Verification items for this drawing (mm, ordinates from the low corner). Give positions to 0.01 mm unless a question says otherwise; leave off trailing zeros. Write each loop counter-clockwise with the first axis right and the second up, starting at its lowest first coordinate (ties: lowest second). Pieces come first, ordered by that corner, then holes. Notation, with made-up numbers: (84, 16) -> (93, 16) arc R25 cw to (93, 30) -> close; hole circle Ø6 at (-4.75, -0.5). An arc over 180 degrees is marked (long way). Use one line per item in the form item = value. Start each with the question number.
(1) Scan lines: L1, parallel to Z at x = 24.25, y = 15; L2, parallel to Y at x = 27, z = 432; L3, parallel to Z at x = 7.5, y = 16 (1 decimal). Record each from-to range of solid material in increasing order.
(2) Section check B-B, the plane x = 6.25. State how many separate pieces and enclosed holes the cut face has, plus the area to 3 significant figures.
(3) Depth check by flat-ended pin: pin 1 Ø1 at (y, z) = (20.5, 320.5) entering from -X. Enter the tip coordinate at first touch or a pass-through.
(4) Section check A-A, the plane z = 77. Record the cut outline in (x, y), plus the area to 3 significant figures.
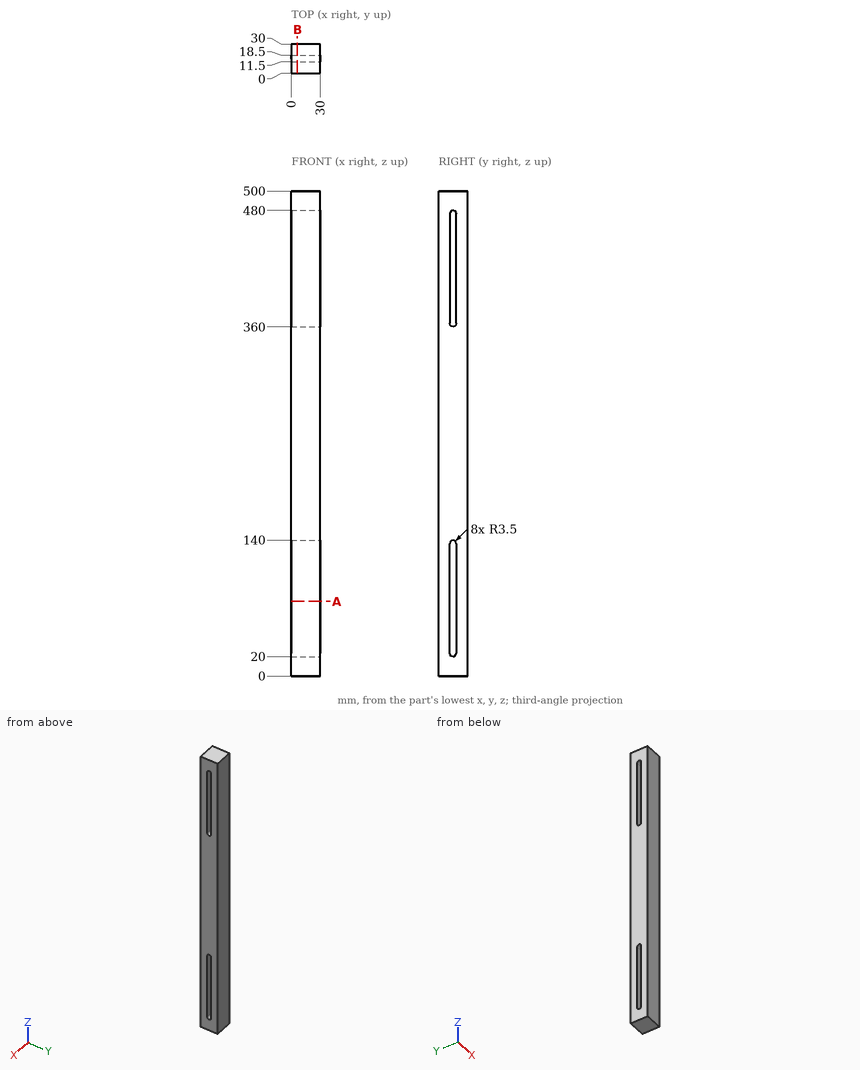
Completed:
q1.L1 = 0 to 20, 140 to 360, 480 to 500
q1.L2 = 0 to 11.5, 18.5 to 30
q1.L3 = 0 to 20.1, 139.9 to 360.1, 479.9 to 500
q2.separate_pieces = 1
q2.enclosed_holes = 2
q2.area = 13,300 mm²
q3.pin_1 = 0
q4.outline = (0, 0) -> (30, 0) -> (30, 11.5) -> (0, 11.5) -> close; (0, 18.5) -> (30, 18.5) -> (30, 30) -> (0, 30) -> close
q4.area = 690 mm²
